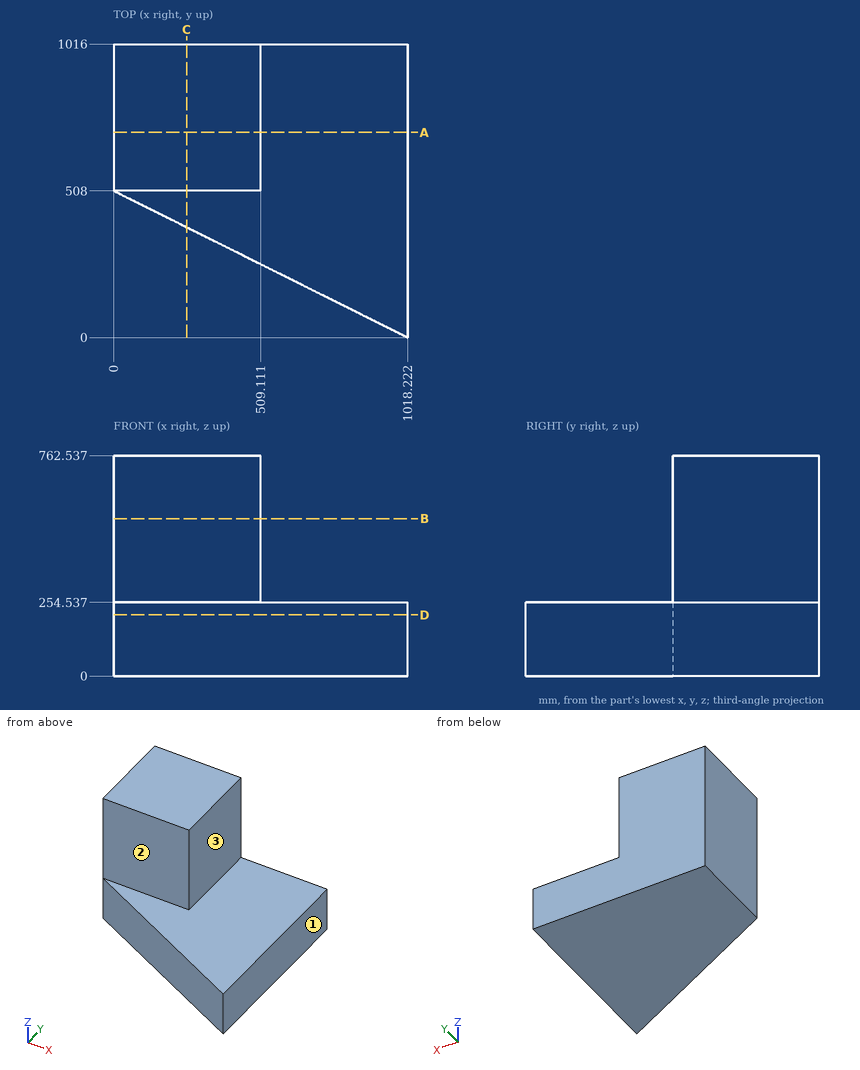
Study the drawing (mm; zero at the part's minimum x, y, z) and answer. A direction names the side the tool comes from. Give positions to 0.01 mm unless a question says otherwise; leave off trailing zeros. Loops run counter-clockwise (first coordinate to the right, second up) from the corner with the lowest first, then second, coordinate; pieces in that order, holes last. Notation, with made-up numbers: M -15.5,75.25 L 33.5,75.25 A16 cw 33.5,94.25 Z; hole C 37,44 d4. An arc over 180 degrees is marked long. Answer as CSV lines item,"result".
Item 1: The part is cut by section C-C (x = 252.5). Give the vertices of the cut face in (y, z) (1 decimal), and give its area (3 significant figures).
Values follow:
outline,"M 382,0 L 1016,0 L 1016,762.5 L 508,762.5 L 508,254.5 L 382,254.5 Z"
area,"419,000 mm^2"
Item 2: Straight lines are drawn through the part: line 1 along X through (y, z) = (527.5, 563.5); line 2 along Z through (x, y) = (834, 584); line 3 along Y through (x, z) = (380.5, 280). For each, find the intervals that lie inside material, in ascending order. Write a range as [from, to].
Values follow:
line 1,"x = [0, 509.11]"
line 2,"z = [0, 254.54]"
line 3,"y = [508, 1016]"
Item 3: Given pin 1 Ø1.5 at (x, z) = (402, 249) entering from -Y (1 decimal); pin 2 Ø10 at (x, y) = (474, 476.5) entering from +Z, each flat-ended and moving along its own axis, determine where each tip first touches the part or whether it passes through.
Values follow:
pin 1,"stops at y = 307.1"
pin 2,"stops at z = 254.54"
Item 4: The part is cut by section B-B (z = 544.5). Give the vertices of the cut face in (x, y).
Values follow:
outline,"M 0,508 L 509.11,508 L 509.11,1016 L 0,1016 Z"
Item 5: The part is cut by section A-A (y = 710). Give the vertices of the cut face in (x, z), and give its area (3 significant figures).
Values follow:
outline,"M 0,0 L 1018.22,0 L 1018.22,254.54 L 509.11,254.54 L 509.11,762.54 L 0,762.54 Z"
area,"518,000 mm^2"
Item 6: Which of the six approach directions +Z, -Z, +X, -X, +Y, -Y give full straight-line access (tool end or side, diameter ignored) to the marked faces 1, 2 and 3?
Values follow:
face 1,"+Z, -Z, +X, +Y, -Y"
face 2,"+Z, +X, -X, -Y"
face 3,"+Z, +X, +Y, -Y"
Item 7: The part is cut by section D-D (z = 211.5). Give the vertices of the cut face in (x, y).
Values follow:
outline,"M 0,508 L 1018.22,0 L 1018.22,1016 L 0,1016 Z"
